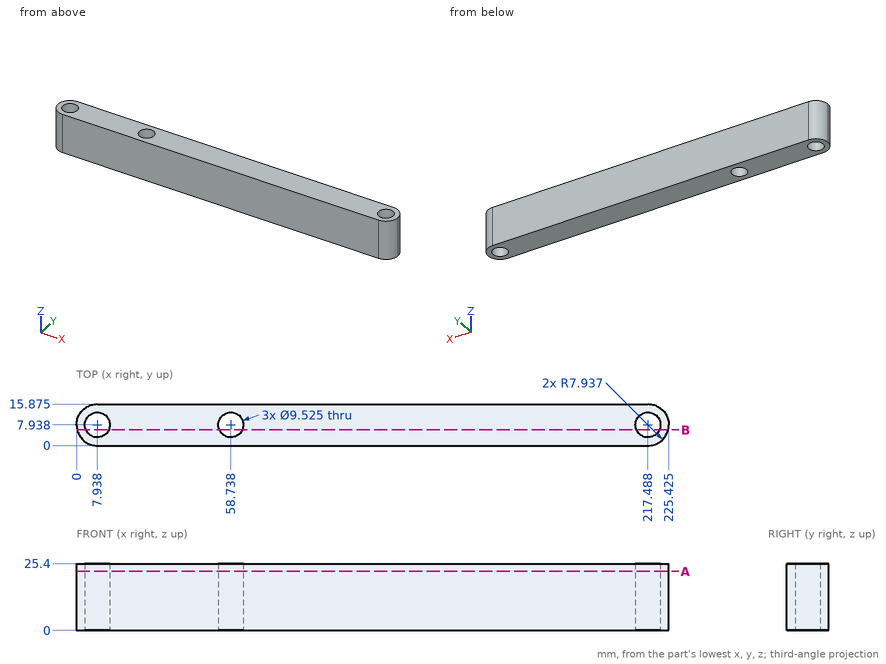
Design review of the part shown in the three views and the two pictorial views. Dimensions are in mm from the part's minimum x, y and z. Give positions to 0.01 mm unless a question says otherwise; leave off trailing zeros. Loops run counter-clockwise (first coordinate to the right, second up) from the corner with the lowest first, then second, coordinate; pieces in that order, holes last. Notation, with made-up numbers: (-7.75, 83.25) -> (26.25, 83.25) arc R36 cw to (26.25, 117.25) -> close; hole circle Ø5 at (18.5, 14). An arc over 180 degrees is marked (long way). Answer as a JSON object with one key per item and string values. Group by question number.
Q1. Take a section at B-B (y = 6). Write out the cut boundary in (x, z) (1 decimal), plus the area to 3 significant figures.
Q2. Take a section at A-A (z = 22.5). State how many separate pieces and enclosed holes the cut face has, plus the area to 3 significant figures.
Q3. Insertion check: pin 1 (1.5 mm diameter, centred on x = 92, y = 4, fed in from -Z); pin 2 (1 mm diameter, centred on y = 6, z = 16, fed in from +X); pin 3 (7.5 mm diameter, centred on x = 217.49, y = 7.94, fed in from +Z). Each pin has a flat end and moves straight along its axis. Give the tip position at first contact, or say it passes through.
Q4. Wall thickness on line 1 along X through (y, z) = (7.5, 18) (1 decimal); line 2 along X through (y, z) = (10, 4) (1 decimal); line 3 along Y through (x, z) = (55, 3.5) (1 decimal): over which ranges is each line inside the solid? List them lowest first.
Answer below:
{
 "1": {"outline": "(0.2, 0) -> (3.6, 0) -> (3.6, 25.4) -> (0.2, 25.4) -> close; (12.3, 0) -> (54.4, 0) -> (54.4, 25.4) -> (12.3, 25.4) -> close; (63.1, 0) -> (213.1, 0) -> (213.1, 25.4) -> (63.1, 25.4) -> close; (221.8, 0) -> (225.2, 0) -> (225.2, 25.4) -> (221.8, 25.4) -> close", "area": "5,050 mm2"},
 "2": {"separate pieces": "1", "enclosed holes": "3", "area": "3,310 mm2"},
 "3": {"pin 1": "stops at z = 0", "pin 2": "stops at x = 225.29", "pin 3": "passes through"},
 "4": {"line 1": "x = 0 to 3.2, 12.7 to 54, 63.5 to 212.7, 222.2 to 225.4", "line 2": "x = 0.3 to 3.6, 12.2 to 54.4, 63 to 213.2, 221.8 to 225.2", "line 3": "y = 0 to 5, 10.9 to 15.9"}
}
